Could you check a few things on this model? Use its own coordinates, in mm. A direction names the side the tool comes from. Round coordinates to 2 decimals unless told otherwise and drop trailing zeros. Loops run counter-clockwise (first coordinate to the right, second up) from the corner with the lowest first, then second, coordinate; pieces in that order, holes last. Notation, with made-up numbers: M 48.5,51 L 64.5,51 A35 cw 64.5,86 Z; hole C 29.5,15.25 d10. An arc over 180 degrees is marked long. Return JSON: item names as keys, results as strings. Group by question number.
```python
from build123d import *

# Parameters (mm, degrees)
CROQUIS1_W                   = 45
CROQUIS1_H                   = 80
CROQUIS1_R                   = 3.25
SALIENTE_EXTRUIR1_DEPTH      = 7
CROQUIS2_R                   = 6.5
CORTAR_EXTRUIR1_DEPTH        = 5
CROQUIS3_R                   = 6
CORTAR_EXTRUIR2_DEPTH        = 0.5
REDONDEO2_R                  = 3
SALIENTE_EXTRUIR2_DEPTH      = 5
TALADROAVANZADO1_OUTLINE_R   = 1.2
TALADROAVANZADO1_DEPTH       = 1
TALADROAVANZADO1_DRAFT       = -45
TALADROAVANZADO1_2_OUTLINE_R = 1.2
TALADROAVANZADO1_2_DEPTH     = 1
TALADROAVANZADO1_2_DRAFT     = -45
CROQUIS8_R                   = 1.2
CORTAR_EXTRUIR3_DEPTH        = 83.006097334
CROQUIS9_W                   = 3
CROQUIS9_H                   = 10
CROQUIS9_R                   = 1
SALIENTE_EXTRUIR3_DEPTH      = 30
CROQUIS10_W                  = 15
CROQUIS10_H                  = 10
SALIENTE_EXTRUIR4_DEPTH      = 3
CROQUIS11_R                  = 1
CORTAR_EXTRUIR5_DEPTH        = 2


# Read off the part's stored shape, not the designer's step: TaladroAvanzado1
with BuildPart() as part:
    # Croquis1 → Saliente-Extruir1 (new body)
    with BuildSketch(Plane.XY):
        Rectangle(CROQUIS1_W, CROQUIS1_H)
        with Locations((5, 20)):
            Circle(CROQUIS1_R, mode=Mode.SUBTRACT)
    extrude(amount=SALIENTE_EXTRUIR1_DEPTH)

    # Croquis2 → Cortar-Extruir1 (cut)
    with BuildSketch(Plane(origin=(0, 0, 0), x_dir=(-1, 0, 0), z_dir=(0, 0, -1))):
        with Locations((-5, 20)):
            Circle(CROQUIS2_R)
    extrude(amount=-CORTAR_EXTRUIR1_DEPTH, mode=Mode.SUBTRACT)

    # Croquis3 → Cortar-Extruir2 (cut)
    with BuildSketch(Plane(origin=(0, 0, 5), x_dir=(-1, 0, 0), z_dir=(0, 0, -1))):
        with Locations((-5, 20)):
            Circle(CROQUIS3_R)
    extrude(amount=-CORTAR_EXTRUIR2_DEPTH, mode=Mode.SUBTRACT)

    # Redondeo2
    redondeo2_edges = [part.edges().sort_by_distance(p)[0] for p in [
        (-22.5, 40, 3.5),
        (22.5, 40, 3.5),
        (22.5, 0, 7),
        (0, 40, 7),
        (-22.5, 0, 7),
        (-22.5, 0, 0),
        (0, 40, 0),
        (22.5, 0, 0),
    ]]
    fillet(redondeo2_edges, radius=REDONDEO2_R)

    # Croquis4 → Saliente-Extruir2 (add)
    with BuildSketch(Plane.XZ.offset(40)):
        with BuildLine():
            Line((-19.5, 7), (-26.5, 7))
            ThreePointArc((-26.5, 7), (-30, 3.5), (-26.5, 0))
            Line((-26.5, 0), (-19.5, 0))
            Line((-19.5, 0), (-19.5, 7))
        make_face()
        with BuildLine():
            Line((19.5, 7), (26.5, 7))
            ThreePointArc((26.5, 7), (30, 3.5), (26.5, 0))
            Line((26.5, 0), (19.5, 0))
            Line((19.5, 0), (19.5, 7))
        make_face()
    extrude(amount=-SALIENTE_EXTRUIR2_DEPTH)


with BuildPart() as taladroavanzado1_tool:
    # TaladroAvanzado1 outline → TaladroAvanzado1 (with draft: the straight prism first)
    with BuildSketch(Plane(origin=(0, -36, 0), x_dir=(1, 0, 0), z_dir=(0, 1, 0))):
        with Locations((26.5, -3.5)):
            Circle(TALADROAVANZADO1_OUTLINE_R)
    extrude(amount=TALADROAVANZADO1_DEPTH)
    # TaladroAvanzado1: the draft: its side faces are tilted about the plane it starts from
    taladroavanzado1_sides = [taladroavanzado1_tool.faces().sort_by_distance(p)[0] for p in [
        (25.3, -35.5, 3.5),
    ]]
    draft(taladroavanzado1_sides, Plane(origin=(0, -36, 0), x_dir=(1, 0, 0), z_dir=(0, 1, 0)), TALADROAVANZADO1_DRAFT)


with BuildPart() as part_1:
    add(part.part)

    # TaladroAvanzado1: cut by taladroavanzado1_tool
    add(taladroavanzado1_tool.part, mode=Mode.SUBTRACT)


with BuildPart() as taladroavanzado1_2_tool:
    # TaladroAvanzado1 2 outline → TaladroAvanzado1 2 (with draft: the straight prism first)
    with BuildSketch(Plane(origin=(0, -36, 0), x_dir=(1, 0, 0), z_dir=(0, 1, 0))):
        with Locations((-26.5, -3.5)):
            Circle(TALADROAVANZADO1_2_OUTLINE_R)
    extrude(amount=TALADROAVANZADO1_2_DEPTH)
    # TaladroAvanzado1 2: the draft: its side faces are tilted about the plane it starts from
    taladroavanzado1_2_sides = [taladroavanzado1_2_tool.faces().sort_by_distance(p)[0] for p in [
        (-27.7, -35.5, 3.5),
    ]]
    draft(taladroavanzado1_2_sides, Plane(origin=(0, -36, 0), x_dir=(1, 0, 0), z_dir=(0, 1, 0)), TALADROAVANZADO1_2_DRAFT)


with BuildPart() as part_2:
    add(part_1.part)

    # TaladroAvanzado1 2: cut by taladroavanzado1_2_tool
    add(taladroavanzado1_2_tool.part, mode=Mode.SUBTRACT)

    # Croquis8 → Cortar-Extruir3 (cut, through all)
    with BuildSketch(Plane(origin=(0, -36, 0), x_dir=(1, 0, 0), z_dir=(0, 1, 0))):
        with Locations(Location((26.5, -3.5, 0), (0, 0, 270))):
            Circle(CROQUIS8_R)
        with Locations(Location((-26.5, -3.5, 0), (0, 0, 270))):
            Circle(CROQUIS8_R)
    extrude(amount=-CORTAR_EXTRUIR3_DEPTH, mode=Mode.SUBTRACT)

    # Croquis9 → Saliente-Extruir3 (add)
    # profile 1 of 2: a face of its own
    with BuildSketch(Plane.XY.offset(7)):
        with Locations((-15, 20)):
            Rectangle(CROQUIS9_W, CROQUIS9_H)
    # profile 2 of 2: a face of its own
    with BuildSketch(Plane.XY.offset(7)):
        with Locations((18, 20)):
            Rectangle(CROQUIS9_W, CROQUIS9_H)
        with Locations((18, 20)):
            Circle(CROQUIS9_R, mode=Mode.SUBTRACT)
    extrude(amount=SALIENTE_EXTRUIR3_DEPTH)

    # Croquis10 → Saliente-Extruir4 (add)
    with BuildSketch(Plane.XY.offset(37)):
        with Locations((-15, 20)):
            Rectangle(CROQUIS10_W, CROQUIS10_H)
        with Locations((18, 20)):
            Rectangle(CROQUIS10_W, CROQUIS10_H)
    extrude(amount=-SALIENTE_EXTRUIR4_DEPTH)

    # Croquis11 → Cortar-Extruir5 (cut)
    with BuildSketch(Plane.XY.offset(37)):
        with Locations((-14.2, 20.567687828)):
            Circle(CROQUIS11_R)
        with Locations((13.55, 20.567687828)):
            Circle(CROQUIS11_R)
    extrude(amount=-CORTAR_EXTRUIR5_DEPTH, mode=Mode.SUBTRACT)


solid = part_2.part
```
1. If we section it at B-B, the plane z = 21: Please give me the cut outline in (x, y), then the cut area to 3 significant figures.
2. On a 3-axis mill with a long thin cutter (end or side, diameter ignored), from which of +Z, -Z, +X, -X, +Y, -Y can I reach the whole of each face in a straight line? I mean faces 5 (the face through (-21.64, 1.5, 0.9)), 6 (the face through (13, 20, 34)), 7 (the face through (-15, 15, 25)). Say none if no direction works.
3. If we section it at C-C, the plane y = -15.5: Please give me the cut outline in (x, z).
4. If we section it at A-A, the plane x = 13.55: Please give me the cut outline in (y, z).
5. We'd pull the mould along Z, two halves only. Please class faces 1 (the face through (-27.565, -37.972, 4.054)), 2 (the face through (18, 20, 34)), 3 (the face through (18, 20, 37)), 4 (the face through (21.6, 39.14, 3.51)): +Z half, -Z half, draft (parallel to the pull), parting line (faces both ways), or undercut.
6. I'm going to push flat-ended pins straight in: pin 1 Ø2.5 at (y, z) = (20.5, 36) entering from +X; pin 2 Ø0.8 at (y, z) = (11.5, 3.5) entering from +X; pin 3 Ø2 at (x, y) = (-10.5, -18) entering from +Z. Where does each tip first touch, or does it pass through?
7. I need wall thicknesses on probe 1 along Y at (x, z) = (5, 3.4); probe 2 along Z at (x, y) = (-11, 18.5); probe 3 along X at (y, z) = (-39, 3). Which ranges of each line are inside material? Lowest first, please.
8. If we section it at D-D, the plane x = -18: Please give me the cut outline in (y, z), then the cut area to 3 significant figures.
Geometry results:
{
 "1": {"outline": "M -16.5,15 L -13.5,15 L -13.5,25 L -16.5,25 Z; M 16.5,15 L 19.5,15 L 19.5,25 L 16.5,25 Z; hole C 18,20 d2", "area": "56.9 mm^2"},
 "2": {"face 5": "-Z, -X, +Y", "face 6": "+Y, -Y", "face 7": "+Z, +X, -X, -Y"},
 "3": {"outline": "M -22.5,3 A3 ccw -19.5,0 L 19.5,0 A3 ccw 22.5,3 L 22.5,4 A3 ccw 19.5,7 L -19.5,7 A3 ccw -22.5,4 Z"},
 "4": {"outline": "M -40,0 L 37,0 A3 ccw 40,3 L 40,4 A3 ccw 37,7 L -40,7 Z; M 15,34 L 25,34 L 25,37 L 21.57,37 L 21.57,35 L 19.57,35 L 19.57,37 L 15,37 Z"},
 "5": {"face 1": "undercut", "face 2": "undercut", "face 3": "+Z half", "face 4": "draft"},
 "6": {"pin 1": "x = 25.5", "pin 2": "x = 22.5", "pin 3": "z = 7"},
 "7": {"probe 1": "-40 to 13.5, 26.5 to 40", "probe 2": "0 to 7, 34 to 37", "probe 3": "-29.96 to -27.59, -25.41 to 25.41, 27.59 to 29.96"},
 "8": {"outline": "M -40,0 L 37,0 A3 ccw 40,3 L 40,4 A3 ccw 37,7 L -40,7 Z; M 15,34 L 25,34 L 25,37 L 15,37 Z", "area": "586 mm^2"}
}
